```python
from build123d import *

# Parameters (mm, degrees)
SKETCH1_W           = 26
SKETCH1_H           = 36
BOSS_EXTRUDE1_DEPTH = 6
SKETCH2_R           = 1.5
BOSS_EXTRUDE2_DEPTH = 10
SKETCH3_R           = 5
SKETCH3_R_2         = 1.5
BOSS_EXTRUDE3_DEPTH = 13


with BuildPart() as part:
    # Sketch1 → Boss-Extrude1 (new body)
    with BuildSketch(Plane(origin=(0, 0, 0), x_dir=(1, 0, 0), z_dir=(0, 1, 0))):
        Rectangle(SKETCH1_W, SKETCH1_H)
    extrude(amount=BOSS_EXTRUDE1_DEPTH)

    # Sketch2 → Boss-Extrude2 (add)
    with BuildSketch(Plane.XY.offset(18)):
        with Locations(Location((0, 3, 0), (0, 0, 180))):
            Circle(SKETCH2_R)
        with Locations(Location((-9, 3, 0), (0, 0, 180))):
            Circle(SKETCH2_R)
        with Locations(Location((9, 3, 0), (0, 0, 180))):
            Circle(SKETCH2_R)
    extrude(amount=BOSS_EXTRUDE2_DEPTH)

    # Sketch3 → Boss-Extrude3 (add)
    with BuildSketch(Plane(origin=(0, 0, -18), x_dir=(-1, 0, 0), z_dir=(0, 0, -1))):
        with Locations(Location((0, 3, 0), (0, 0, 143.130102354))):
            Circle(SKETCH3_R)
        with Locations(Location((-11, 3, 0), (0, 0, 180))):
            Circle(SKETCH3_R_2)
        with Locations(Location((11, 3, 0), (0, 0, 180))):
            Circle(SKETCH3_R_2)
    extrude(amount=BOSS_EXTRUDE3_DEPTH)


solid = part.part
```
The listing builds one solid part. Answer for the finished solid, in the listing's coordinates (mm). A direction names the side the tool comes from. Give positions to 0.01 mm unless a question says otherwise; leave off trailing zeros. Order: outer loops, then holes, each group sorted by start corner. A loop starts at its lowest first (then second) coordinate and runs counter-clockwise, first axis right, second up. Notation, with made-up numbers: (41.5, 59.5) -> (73.5, 59.5) arc R21 cw to (73.5, 75.5) -> close; hole circle Ø4 at (6.25, 31). An arc over 180 degrees is marked (long way). One line per item, written item: value.
1) Determine the mould class of faces 1 (the flat face through (13, 3, 0)), 2 (the cylindrical face through (10.11, 1.99, 22.93)), 3 (the flat face through (0, 0, 0)) for opening direction X: pulls with the +X half, pulls with the -X half, needs draft (parallel to the pull), parting line crosses it, or undercut.
Reported:
face 1: pulls with the +X half
face 2: undercut
face 3: needs draft
2) Find section C-C, the plane z = -15. Determine the outline of the cut face in (x, y), plus the area to 3 significant figures.
Reported:
outline: (-13, 0) -> (13, 0) -> (13, 6) -> (-13, 6) -> close
area: 156 mm^2
3) Find section B-B, the plane y = 3. Determine the outline of the cut face in (x, z), plus the area to 3 significant figures.
Reported:
outline: (-13, -18) -> (-12.5, -18) -> (-12.5, -31) -> (-9.5, -31) -> (-9.5, -18) -> (-5, -18) -> (-5, -31) -> (5, -31) -> (5, -18) -> (9.5, -18) -> (9.5, -31) -> (12.5, -31) -> (12.5, -18) -> (13, -18) -> (13, 18) -> (10.5, 18) -> (10.5, 28) -> (7.5, 28) -> (7.5, 18) -> (1.5, 18) -> (1.5, 28) -> (-1.5, 28) -> (-1.5, 18) -> (-7.5, 18) -> (-7.5, 28) -> (-10.5, 28) -> (-10.5, 18) -> (-13, 18) -> close
area: 1,230 mm^2
4) A tool of negligible diameter and unlimited length cuts with its end or side. For faces 4 (the cylindrical face through (-4, 6, -24)), 5 (the flat face through (0, -1, -18)), 6 (the flat face through (0, 7, -18)), 7 (the cylindrical face through (-7.89, 1.99, 22.93)), from which of +Z, -Z, +X, -X, +Y, -Y can it reach the whole face along a straight path? Write none if from no direction.
Reported:
face 4: -Z
face 5: +Z, +X, -X, -Y
face 6: +Z, +X, -X, +Y
face 7: +Z
5) Find section A-A, the plane x = 0. Determine the outline of the cut face in (y, z), plus the area to 3 significant figures.
Reported:
outline: (-2, -31) -> (8, -31) -> (8, -18) -> (6, -18) -> (6, 18) -> (4.5, 18) -> (4.5, 28) -> (1.5, 28) -> (1.5, 18) -> (0, 18) -> (0, -18) -> (-2, -18) -> close
area: 376 mm^2
6) Find the intervals of material crossed by line 1 (X direction, y = 2, z = -27); line 2 (Y direction, x = 9, z = 9.5); line 3 (Y direction, x = -9, z = 23.5), in increasing order.
Reported:
line 1: x = -12.12 to -9.88, -4.9 to 4.9, 9.88 to 12.12
line 2: y = 0 to 6
line 3: y = 1.5 to 4.5
7) Flat-ended cylindrical pins translate along their axes: P1, Ø1, axis at x = -7.5, z = -12, coming from the -Y side; P2, Ø1.6, axis at x = -2, y = 6.5, coming from the +Z side; P3, Ø4, axis at y = 6.5, z = 13.5, coming from the -X side; P4, Ø1.8, axis at x = -7.5, y = 3, coming from the -Z side. Find the tip coordinate at first contact, or state that the pin passes through.
Reported:
P1: stops at y = 0
P2: stops at z = 18
P3: stops at x = -13
P4: stops at z = -18
